Read the model definition and answer for the solid it produces. Units are mm, in the model's axes. Face numbers are marked on the shaded views. A direction names the side the tool comes from. Coordinates: 2 decimals unless noted, no trailing zeros. Loops run counter-clockwise (first coordinate to the right, second up) from the corner with the lowest first, then second, coordinate; pieces in that order, holes last. Notation, with made-up numbers: (4.5, 57.5) -> (58.5, 57.5) arc R25 ccw to (58.5, 84.5) -> close; hole circle Ø4 at (2, 23). An arc over 180 degrees is marked (long way). Answer as CSV lines item,"result".
```python
from build123d import *

# Parameters (mm, degrees)
F0_R     = 32.5
F0_R_2   = 22.5
F1_DEPTH = 10
F2_DEPTH = 13
F3_DEPTH = 8
F4_R     = 2.99999


# Not quite as in the source:
# - a fillet or chamfer is up to 0.001 mm smaller than in the source, because OpenCascade refuses the exact size


with BuildPart() as f1:
    # F0 (on Top) → F1 (new body)
    with BuildSketch(Plane.XY):
        Circle(F0_R)
        Circle(F0_R_2, mode=Mode.SUBTRACT)
        Circle(F0_R_2)
        Polygon((-8.5, 4.9074772881), (0, 9.8149545762), (8.5, 4.9074772881), (8.5, -4.9074772881), (0, -9.8149545762), (-8.5, -4.9074772881), align=None, mode=Mode.SUBTRACT)
        Polygon((8.5, 4.9074772881), (0, 9.8149545762), (-8.5, 4.9074772881), (-8.5, -4.9074772881), (0, -9.8149545762), (8.5, -4.9074772881), align=None)
    extrude(amount=F1_DEPTH)

    # F0 (on Top) → F2 (join)
    with BuildSketch(Plane.XY):
        Circle(F0_R)
        Circle(F0_R_2, mode=Mode.SUBTRACT)
    extrude(amount=F2_DEPTH)

    # F0 (on Top) → F3 (cut)
    with BuildSketch(Plane.XY):
        Polygon((8.5, 4.9074772881), (0, 9.8149545762), (-8.5, 4.9074772881), (-8.5, -4.9074772881), (0, -9.8149545762), (8.5, -4.9074772881), align=None)
    extrude(amount=F3_DEPTH, mode=Mode.SUBTRACT)

    # F4 (radius 3 in the source; OpenCascade refuses exactly that, so slightly less here)
    f4_edges = [f1.edges().sort_by_distance(p)[0] for p in [
        (-32.5, 0, 13),
        (-22.5, 0, 13),
    ]]
    fillet(f4_edges, radius=F4_R)


solid = f1.part
```
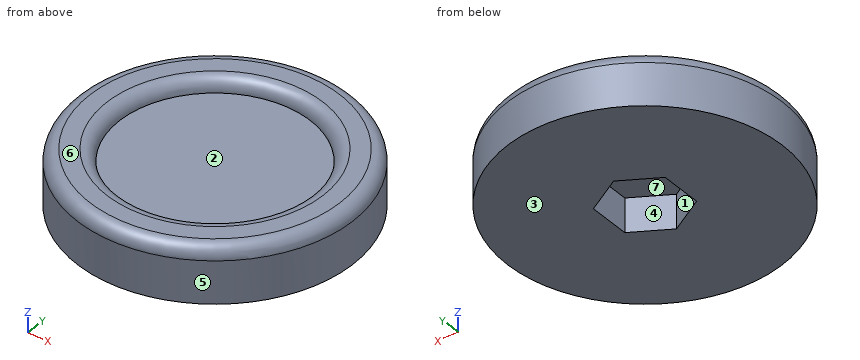
Q1. For the marked faces 1, 2 and 3, determine the directions among +Z, -Z, +X, -X, +Y, -Y from which every point of the face is accessible in a straight line to the end or side of a thin tool.
Results:
face 1,"-Z"
face 2,"+Z"
face 3,"-Z, +X, -X, +Y, -Y"
Q2. A cutting plane is placed at C-C, the plane z = 9. Write down the section's boundary in (x, y).
Results:
outline,"circle Ø65 at (0, 0)"
Q3. A cutting plane is placed at A-A, the plane z = 2. Write down the section's boundary in (x, y).
Results:
outline,"circle Ø65 at (0, 0); hole (-8.5, -4.91) -> (0, -9.81) -> (8.5, -4.91) -> (8.5, 4.91) -> (0, 9.81) -> (-8.5, 4.91) -> close"
Q4. Given pin 1 Ø6 at (x, z) = (-4, 9) entering from -Y; pin 2 Ø5 at (y, z) = (-3, 4.5) entering from -X; pin 3 Ø2 at (x, y) = (-11, 20) entering from +Z; pin 4 Ø13.5 at (x, y) = (-4, 2.5) entering from -Z, each flat-ended and moving along its own axis, determine where each tip first touches the part or whether it passes through.
Results:
pin 1,"stops at y = -32.48"
pin 2,"stops at x = -32.5"
pin 3,"stops at z = 12.49"
pin 4,"stops at z = 0"
Q5. Find the intervals of material crossed by probe 1 along Y at (x, z) = (0, 10.05); probe 2 along Z at (x, y) = (-10.5, -14); probe 3 along X at (y, z) = (-9, 7.75), in increasing order. Write a range as [from, to].
Results:
probe 1,"y = [-32.5, -22.5], [22.5, 32.5]"
probe 2,"z = [0, 10]"
probe 3,"x = [-31.23, -1.41], [1.41, 31.23]"
Q6. For a pull along Y with two mould halves and no side action, classify the marked faces 4, 5, 6 and 7 as pulls with the +Y half, pulls with the -Y half, needs draft (parallel to the pull), parting line crosses it, or undercut.
Results:
face 4,"undercut"
face 5,"parting line crosses it"
face 6,"needs draft"
face 7,"undercut"
